from build123d import *

# Parameters (mm, degrees)
SKETCH1_W           = 60
SKETCH1_H           = 60
SKETCH1_R           = 2.2
BOSS_EXTRUDE1_DEPTH = 19
SKETCH2_R           = 11
CUT_EXTRUDE1_DEPTH  = 4
CUT_EXTRUDE2_REACH  = 58
SKETCH3_R           = 5.2
SKETCH4_R           = 7.2
CUT_EXTRUDE3_DEPTH  = 46
SKETCH5_R           = 1.3
CUT_EXTRUDE4_DEPTH  = 6
SKETCH6_R           = 7.071067812
CUT_EXTRUDE5_DEPTH  = 5


with BuildPart() as part:
    # Sketch1 → Boss-Extrude1 (new body)
    with BuildSketch(Plane.XY):
        Rectangle(SKETCH1_W, SKETCH1_H)
        with Locations((-25, 25)):
            Circle(SKETCH1_R, mode=Mode.SUBTRACT)
        with Locations((25, 25)):
            Circle(SKETCH1_R, mode=Mode.SUBTRACT)
        with Locations((25, -25)):
            Circle(SKETCH1_R, mode=Mode.SUBTRACT)
        with Locations((-25, -25)):
            Circle(SKETCH1_R, mode=Mode.SUBTRACT)
    extrude(amount=BOSS_EXTRUDE1_DEPTH)

    # Sketch2 → Cut-Extrude1 (cut)
    with BuildSketch(Plane(origin=(0, 30, 0), x_dir=(1, 0, 0), z_dir=(0, 1, 0))):
        with Locations((0, -7.7)):
            Circle(SKETCH2_R)
    extrude(amount=-CUT_EXTRUDE1_DEPTH, mode=Mode.SUBTRACT)

    # Sketch3 → Cut-Extrude2 (cut, up to next)
    with BuildSketch(Plane(origin=(0, 26, 0), x_dir=(1, 0, 0), z_dir=(0, 1, 0)), mode=Mode.PRIVATE) as cut_extrude2_sk1:
        with Locations((0, -7.7)):
            Circle(SKETCH3_R)
    cut_extrude2_tool1 = extrude(cut_extrude2_sk1.sketch, amount=-CUT_EXTRUDE2_REACH, mode=Mode.PRIVATE) & part.part
    add(cut_extrude2_tool1.solids().sort_by_distance((0, 26, 7.7))[0], mode=Mode.SUBTRACT)

    # Sketch4 → Cut-Extrude3 (cut)
    with BuildSketch(Plane.XZ.offset(30)):
        with Locations((0, 7.7)):
            Circle(SKETCH4_R)
    extrude(amount=-CUT_EXTRUDE3_DEPTH, mode=Mode.SUBTRACT)

    # Sketch5 → Cut-Extrude4 (cut)
    with BuildSketch(Plane(origin=(0, 26, 0), x_dir=(1, 0, 0), z_dir=(0, 1, 0))):
        with Locations((-5.303300859, -2.396699141)):
            Circle(SKETCH5_R)
        with Locations((5.303300859, -2.396699141)):
            Circle(SKETCH5_R)
        with Locations((5.303300859, -13.003300859)):
            Circle(SKETCH5_R)
        with Locations((-5.303300859, -13.003300859)):
            Circle(SKETCH5_R)
    extrude(amount=-CUT_EXTRUDE4_DEPTH, mode=Mode.SUBTRACT)

    # Sketch6 → Cut-Extrude5 (cut)
    with BuildSketch(Plane(origin=(0, 0, 0), x_dir=(-1, 0, 0), z_dir=(0, 0, -1))):
        with Locations((-25, 25)):
            Circle(SKETCH6_R)
        with Locations((25, 25)):
            Circle(SKETCH6_R)
        with Locations((25, -25)):
            Circle(SKETCH6_R)
        with Locations((-25, -25)):
            Circle(SKETCH6_R)
    extrude(amount=-CUT_EXTRUDE5_DEPTH, mode=Mode.SUBTRACT)


solid = part.part
Here's how the part is built. I have some questions about the finished solid (model axes, mm). A direction names the side the tool comes from. Coordinates: 2 decimals unless noted, no trailing zeros. Loops run counter-clockwise (first coordinate to the right, second up) from the corner with the lowest first, then second, coordinate; pieces in that order, holes last.
1. Imagine slicing it at C-C, the plane y = -16. Please give me the cut outline in (x, z).
2. For faces 4 (the cylindrical face through (-0.94, -7.32, 14.84)), 5 (the cylindrical face through (20, -20, 2)), 6 (the cylindrical face through (-6.6, 23, 2.3)), 7 (the cylindrical face through (24.523, 22.852, 11.902)), which set-ups out of +Z, -Z, +X, -X, +Y, -Y let a thin tool reach every point of the face, with its end or its side?
3. Imagine slicing it at B-B, the plane x = 25. Please give me the cut outline in (y, z), and give its area (3 significant figures).
4. If we mould it in two halves opening along X, with no side actions, what happens to faces 1 (the cylindrical face through (-0.677, 21.07, 2.544)), 2 (the flat face through (0, 0, 19)), 3 (the flat face through (-30, 0, 9))? For each: pulls with the +X half, pulls with the -X half, needs draft (parallel to the pull), parting line crosses it, or undercut.
5. For P1, Ø7, axis at x = -25, y = 25, coming from the -Z side; P2, Ø1.3, axis at x = 4.5, z = 12.5, coming from the +Y side; P3, Ø2.5, axis at x = -5.3, z = 13, coming from the +Y side, each with a flat end and sliding along its axis, tell me the tip position at first contact or that it passes through.
6. Imagine slicing it at D-D, the plane x = 3. Please give me the cut outline in (y, z), and give its area (3 significant figures).
7. I need wall thicknesses on L1, parallel to Y at x = -25, z = 16; L2, parallel to Z at x = 5.5, y = 22; L3, parallel to Z at x = 0.5, y = -18.5. Which ranges of each line are inside material? Lowest first, please.
8. Imagine slicing it at A-A, the plane z = 7.7. Please give me the cut outline in (x, y).
Taken from the geometry:
1. outline: (-30, 0) - (30, 0) - (30, 19) - (-30, 19) - close; hole circle Ø14.4 at (0, 7.7)
2. face 4: -Y
2. face 5: -Z
2. face 6: +Y
2. face 7: +Z, -Z
3. outline: (-30, 5) - (-27.2, 5) - (-27.2, 19) - (-30, 19) - close; (-22.8, 5) - (-17.93, 5) - (-17.93, 0) - (17.93, 0) - (17.93, 5) - (22.8, 5) - (22.8, 19) - (-22.8, 19) - close; (27.2, 5) - (30, 5) - (30, 19) - (27.2, 19) - close
3. area: 896 mm2
4. face 1: undercut
4. face 2: needs draft
4. face 3: pulls with the -X half
5. P1: stops at z = 5
5. P2: stops at y = 26
5. P3: stops at y = 20
6. outline: (-30, 0) - (26, 0) - (26, 3.45) - (16, 3.45) - (16, 1.15) - (-30, 1.15) - close; (-30, 14.25) - (16, 14.25) - (16, 11.95) - (26, 11.95) - (26, 18.28) - (30, 18.28) - (30, 19) - (-30, 19) - close
6. area: 380 mm2
7. L1: y = -30 to -27.2, -22.8 to 22.8, 27.2 to 30
7. L2: z = 0 to 1.11, 3.68 to 11.72, 14.29 to 19
7. L3: z = 0 to 0.52, 14.88 to 19
8. outline: (-30, -30) - (-7.2, -30) - (-7.2, 16) - (-5.2, 16) - (-5.2, 26) - (-11, 26) - (-11, 30) - (-30, 30) - close; (5.2, 16) - (7.2, 16) - (7.2, -30) - (30, -30) - (30, 30) - (11, 30) - (11, 26) - (5.2, 26) - close; hole circle Ø4.4 at (-25, -25); hole circle Ø4.4 at (-25, 25); hole circle Ø4.4 at (25, -25); hole circle Ø4.4 at (25, 25)
